```python
from build123d import *

# Parameters (mm, degrees)
F1_DEPTH = 2.54
F2_DEPTH = 2.794
F5_DEPTH = 2.54


# Not quite as in the source:
# - ends of sketch curves that miss each other by under 0.0002 mm in the source are joined


with BuildPart() as f1:
    # F0 (on Top) → F1 (new body)
    with BuildSketch(Plane.XY):
        Polygon((40.704589831, -14.0446320264), (45.6521262704, -14.1146421426), (31.6115576886, 3.3264026483), (26.7203815156, 3.3264026483), (24.2085343305, 6.4465921843), (-38.9784165732, 6.4465921843), (-22.1132018277, -19.5065848529), (45.1016274707, -19.5065848529), (43.1621550999, -17.0973931503), align=None)
        Polygon((26.7203815156, 3.3264026483), (31.6115576886, 3.3264026483), (26.0325449788, 10.2565921843), (-41.4542779326, 10.2565921843), (-38.9784165732, 6.4465921843), (24.2085343305, 6.4465921843), align=None)
        Polygon((53.0599689064, -23.3165845275), (49.0268522152, -18.3066903858), (45.6521262704, -14.1146421426), (40.704589831, -14.0446320264), (43.1621550999, -17.0973931503), (45.1016274707, -19.5065848529), (-22.1132018277, -19.5065848529), (-19.6373406798, -23.3165845275), align=None)
    extrude(amount=-F1_DEPTH)

    # F0 (on Top) → F2 (join)
    with BuildSketch(Plane.XY):
        Polygon((26.7203815156, 3.3264026483), (31.6115576886, 3.3264026483), (26.0325449788, 10.2565921843), (-41.4542779326, 10.2565921843), (-38.9784165732, 6.4465921843), (24.2085343305, 6.4465921843), align=None)
        Polygon((53.0599689064, -23.3165845275), (49.0268522152, -18.3066903858), (45.6521262704, -14.1146421426), (40.704589831, -14.0446320264), (43.1621550999, -17.0973931503), (45.1016274707, -19.5065848529), (-22.1132018277, -19.5065848529), (-19.6373406798, -23.3165845275), align=None)
    extrude(amount=F2_DEPTH)

    # F4 (on offset) → F5 (join)
    with BuildSketch(Plane.XY.offset(2.794)):
        Polygon((53.0598776368, -23.3175773174), (49.0267609456, -18.3076831757), (45.6520350008, -14.1156349324), (40.7044985614, -14.0456248163), (43.1620638303, -17.0983859402), (45.101536201, -19.5075776428), (-22.1132930973, -19.5075776428), (-19.6374319494, -23.3175773174), align=None)
        Polygon((40.7044985614, -14.0456248163), (45.6520350008, -14.1156349324), (31.611466419, 3.3254098585), (26.720290246, 3.3254098585), (24.2084430609, 6.4455993944), (-38.9785078428, 6.4455993944), (-22.1132930973, -19.5075776428), (45.101536201, -19.5075776428), (43.1620638303, -17.0983859402), align=None)
        Polygon((26.720290246, 3.3254098585), (31.611466419, 3.3254098585), (26.0324537092, 10.2555993944), (-41.4543692023, 10.2555993944), (-38.9785078428, 6.4455993944), (24.2084430609, 6.4455993944), align=None)
    extrude(amount=F5_DEPTH)


solid = f1.part
```
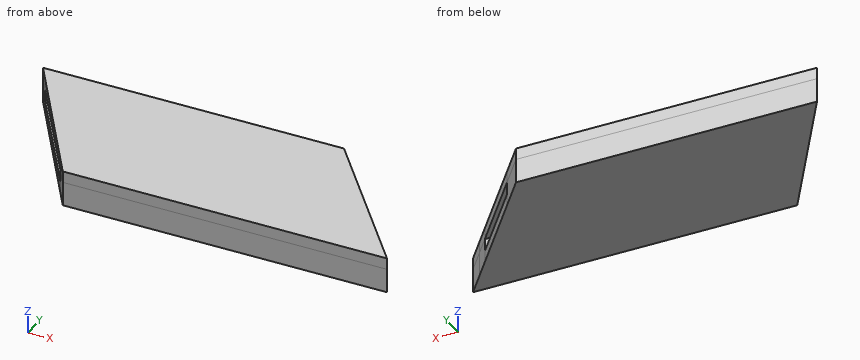
Input: part model. Units: mm. Frame: model coordinates. Coordinates: 2 decimals unless noted, no trailing zeros. Loops run counter-clockwise (first coordinate to the right, second up) from the corner with the lowest first, then second, coordinate; pieces in that order, holes last.
Q1. Section B-B, the plane z = 1. Return the cut outline in (x, y), and give its area (3 significant figures).
Results are:
outline: (-41.45, 10.26) - (-38.98, 6.45) - (24.21, 6.45) - (26.72, 3.33) - (31.61, 3.33) - (26.03, 10.26) - close; (-22.11, -19.51) - (-19.64, -23.32) - (53.06, -23.32) - (45.65, -14.11) - (40.7, -14.04) - (45.1, -19.51) - close
area: 576 mm2
Q2. Section C-C, the plane y = 1. Return the cut outline in (x, z).
Results are:
outline: (-35.44, -2.54) - (33.48, -2.54) - (33.48, 0) - (-35.44, 0) - close; (-35.44, 2.79) - (33.48, 2.79) - (33.48, 5.33) - (-35.44, 5.33) - close
Q3. Section D-D, the plane y = -5. Return the cut outline in (x, z).
Results are:
outline: (-31.54, -2.54) - (38.31, -2.54) - (38.31, 0) - (-31.54, 0) - close; (-31.54, 2.79) - (38.31, 2.79) - (38.31, 5.33) - (-31.54, 5.33) - close
Q4. Line query: line 1 along Z through (x, y) = (0.5, -7); line 2 along Y through (x, z) = (-12.5, 1.75); line 3 along Y through (x, z) = (-23, 1.5). Output: solid intervals per line, ascending.
Results are:
line 1: z = -2.54 to 0, 2.79 to 5.33
line 2: y = -23.32 to -19.51, 6.45 to 10.26
line 3: y = 6.45 to 10.26
Q5. Contact query for flat-ended pins moving along their axis: pin 1 (1.5 mm diameter, centred on y = 2.5, z = -1, fed in from +X); pin 2 (1.5 mm diameter, centred on y = 1, z = 2.5, fed in from -X). Output: stop coordinate, or through.
Results are:
pin 1: stops at x = 32.88
pin 2: stops at x = -35.89
